Geometry: see drawing. Coordinates: mm, zero at the bounding-box minimum. Coordinates: 2 decimals unless noted, no trailing zeros. Order: outer loops, then holes, each group sorted by start corner. A loop starts at its lowest first (then second) coordinate and runs counter-clockwise, first axis right, second up.
Item 1: Section C-C on z = 73. Return the cut outline in (x, y).
Item 2: Section B-B on x = 24.75. Return the cut outline in (y, z), then the cut area to 3 significant figures.
Item 3: Ray query, line 1 (Z direction, x = 10, y = 24); line 2 (Y direction, x = 13, z = 16); line 3 (Y direction, x = 14, z = 72). Return the intervals inside material, ascending.
Item 4: Section A-A on y = 14.25. Return the cut outline in (x, z).
Item 5: Section D-D on x = 8.5. Return the cut outline in (y, z).
Item 6: Contact query for flat-ended pins moving along their axis: P1, Ø10, axis at x = 4.5, y = 21.5, coming from the -Z side; P2, Ø1, axis at y = 22, z = 54.5, coming from the +X side; P3, Ø5, axis at y = 17, z = 62.5, coming from the -X side; P4, Ø1.5, axis at x = 18, z = 39.5, coming from the -Y side. Output: stop coordinate, or through.
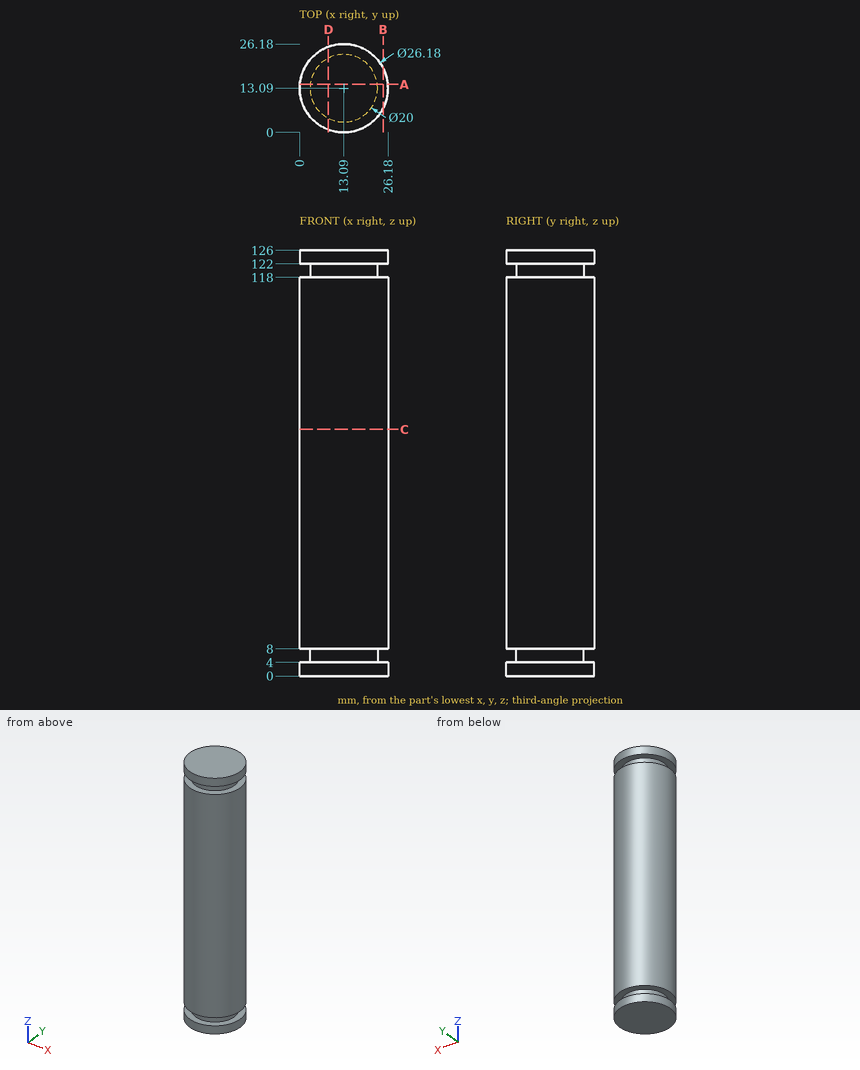
Answer list:
1. outline: circle Ø26.18 at (13.09, 13.09)
2. outline: (7.14, 0) - (19.04, 0) - (19.04, 4) - (7.14, 4) - close; (7.14, 8) - (19.04, 8) - (19.04, 118) - (7.14, 118) - close; (7.14, 122) - (19.04, 122) - (19.04, 126) - (7.14, 126) - close
2. area: 1,400 mm2
3. line 1: z = 0 to 4, 8 to 118, 122 to 126
3. line 2: y = 0 to 26.18
3. line 3: y = 0.03 to 26.15
4. outline: (0.05, 0) - (26.13, 0) - (26.13, 4) - (23.02, 4) - (23.02, 8) - (26.13, 8) - (26.13, 118) - (23.02, 118) - (23.02, 122) - (26.13, 122) - (26.13, 126) - (0.05, 126) - (0.05, 122) - (3.16, 122) - (3.16, 118) - (0.05, 118) - (0.05, 8) - (3.16, 8) - (3.16, 4) - (0.05, 4) - close
5. outline: (0.83, 0) - (25.35, 0) - (25.35, 4) - (21.97, 4) - (21.97, 8) - (25.35, 8) - (25.35, 118) - (21.97, 118) - (21.97, 122) - (25.35, 122) - (25.35, 126) - (0.83, 126) - (0.83, 122) - (4.21, 122) - (4.21, 118) - (0.83, 118) - (0.83, 8) - (4.21, 8) - (4.21, 4) - (0.83, 4) - close
6. P1: stops at z = 0
6. P2: stops at x = 23.12
6. P3: stops at x = 0.08
6. P4: stops at y = 0.68
